The model under review builds one solid part; all positions refer to its coordinate system, in mm. A direction names the side the tool comes from. Coordinates: 2 decimals unless noted, no trailing zeros. Write each loop counter-clockwise with the first axis right and the second up, starting at its lowest first coordinate (ties: lowest second). Pieces come first, ordered by that corner, then holes.
1) Add section A-A, the plane x = 0. State the section outline as (y, z) points, then the cut area to 3 significant figures.
2) Machinability: for faces 1 (the cylindrical face through (-19.43, -3.17, 0.53)), 2 (the cylindrical face through (0.279, -12.697, -44.361)), 3 (the flat face through (-28, -6.35, 1)), which of the approach directions +Z, -Z, +X, -X, +Y, -Y give a long, thin tool a straight path to every point of the face, cutting with its end or side? Answer none if there is none.
3) For P1, Ø11, axis at x = -28.575, z = -22.225, coming from the +Y side; P2, Ø12, axis at x = -26.5, z = 1, coming from the -Y side, all flat-tipped, find the tip position at first contact; note any pin that passes through.
4) Add section D-D, the plane z = 42. State the section outline as (x, y) points, then the cut area to 3 significant figures.
5) Add section C-C, the plane y = -10. State the section outline as (x, z) points, then the cut area to 3 significant figures.
6) For line 1 (Z direction, x = -9, y = -12.5); line 2 (Z direction, x = -30, y = -1.25); line 3 (X direction, y = -3, z = 39.5), list the stretches that pass through material, from the lowest coordinate up.
7) Mouldability with a two-part tool opening along Z and no side actions: class faces 4 (the flat face through (-1, -14, -38.1)), 5 (the cylindrical face through (2.853, -18.835, -44.361)), 6 (the flat face through (-10, -9, -50.8)) as released by +Z, released by -Z, zero draft, split by the parting line, or undercut.
8) Add section B-B, the plane y = -4. State the section outline as (x, z) points (1 decimal), then the cut area to 3 significant figures.
from build123d import *

# Parameters (mm, degrees)
F1_DEPTH = 50.8
F2_R     = 19.685
F3_DEPTH = 38.1
F4_R     = 4.7625
F5_DEPTH = 12.7


with BuildPart() as f1:
    # F0 (on Top) → F1 (new body, symmetric)
    with BuildSketch(Plane.XY):
        with BuildLine():
            Line((-12.7, 0), (-38.1, 0))
            Line((-38.1, 0), (-38.1, -6.35))
            Line((-38.1, -6.35), (-17.960512, -6.35))
            ThreePointArc((-17.960512, -6.35), (3.221393, -18.775653), (19.05, 0))
            Line((19.05, 0), (12.7, 0))
            ThreePointArc((12.7, 0), (0, -12.7), (-12.7, 0))
        make_face()
    extrude(amount=F1_DEPTH, both=True)

    # F2 (on Top) → F3 (cut, symmetric)
    with BuildSketch(Plane.XY):
        Circle(F2_R)
    extrude(amount=F3_DEPTH, both=True, mode=Mode.SUBTRACT)

    # F4 (on face) → F5 (cut)
    with BuildSketch(Plane.XZ.offset(6.35)):
        with Locations((-28.575, 22.225)):
            Circle(F4_R)
        with Locations((-28.575, -22.225)):
            Circle(F4_R)
    extrude(amount=-F5_DEPTH, mode=Mode.SUBTRACT)


solid = f1.part
Geometry results:
1. outline: (-19.05, -50.8) - (-12.7, -50.8) - (-12.7, -38.1) - (-19.05, -38.1) - close; (-19.05, 38.1) - (-12.7, 38.1) - (-12.7, 50.8) - (-19.05, 50.8) - close
1. area: 161 mm2
2. face 1: +X, +Y
2. face 2: +Z, -Z, +Y
2. face 3: +Z, -Z, -X, -Y
3. P1: stops at y = 0
3. P2: stops at y = -6.35
4. outline: (-38.1, -6.35) - (-17.96, -6.35) arc R19.05 ccw to (19.05, 0) - (12.7, 0) arc R12.7 cw to (-12.7, 0) - (-38.1, 0) - close
4. area: 440 mm2
5. outline: (-16.21, -50.8) - (-7.83, -50.8) - (-7.83, -38.1) - (-16.21, -38.1) - close; (-16.21, 38.1) - (-7.83, 38.1) - (-7.83, 50.8) - (-16.21, 50.8) - close; (7.83, -50.8) - (16.21, -50.8) - (16.21, -38.1) - (7.83, -38.1) - close; (7.83, 38.1) - (16.21, 38.1) - (16.21, 50.8) - (7.83, 50.8) - close
5. area: 426 mm2
6. line 1: z = -50.8 to -38.1, 38.1 to 50.8
6. line 2: z = -50.8 to -26.77, -17.68 to 17.68, 26.77 to 50.8
6. line 3: x = -38.1 to -12.34, 12.34 to 18.81
7. face 4: undercut
7. face 5: zero draft
7. face 6: released by -Z
8. outline: (-38.1, -50.8) - (-12.1, -50.8) - (-12.1, -38.1) - (-19.3, -38.1) - (-19.3, 38.1) - (-12.1, 38.1) - (-12.1, 50.8) - (-38.1, 50.8) - close; (12.1, -50.8) - (18.6, -50.8) - (18.6, -38.1) - (12.1, -38.1) - close; (12.1, 38.1) - (18.6, 38.1) - (18.6, 50.8) - (12.1, 50.8) - close; hole circle Ø9.5 at (-28.6, -22.2); hole circle Ø9.5 at (-28.6, 22.2)
8. area: 2,120 mm2
